Could you check a few things on this model? Use its own coordinates, in mm. Face numbers are marked on the shaded views. A direction names the side the tool comes from. Coordinates: 2 decimals unless noted, no trailing zeros. Loops run counter-clockwise (first coordinate to the right, second up) from the corner with the lowest first, then second, coordinate; pieces in that order, holes last. Notation, with made-up numbers: (3.25, 53.25) -> (57.25, 53.25) arc R4 ccw to (57.25, 59.25) -> close; hole circle Ø2 at (-36, 63). An arc over 180 degrees is marked (long way). One line per question, with ' | ' between items.
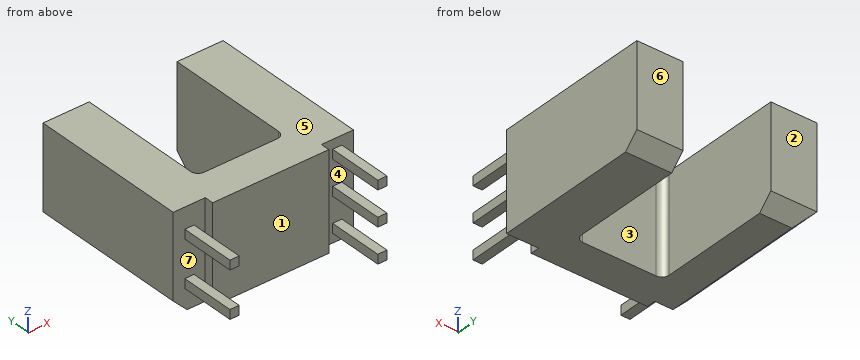
```python
from build123d import *

# Parameters (mm, degrees)
BOSS_EXTRUDE1_DEPTH      = 2.665
CHAMFER1_SIZE            = 0.76
SKETCH2_W                = 1.76
SKETCH2_H                = 5.33
CUT_EXTRUDE1_DEPTH       = 0.5
FILLET1_R                = 0.4
SKETCH3_W                = 0.508
SKETCH3_H                = 0.508
BOSS_EXTRUDE2_DEPTH      = 2.54
BOSS_EXTRUDE2_DEPTH_BACK = 0.5


with BuildPart() as part:
    # Sketch1 → Boss-Extrude1 (new body, symmetric)
    with BuildSketch(Plane.XY):
        Polygon((2.415, 9.27), (4.955, 9.27), (4.955, 0), (-4.955, 0), (-4.955, 9.27), (-2.415, 9.27), (-2.415, 2.03), (2.415, 2.03), align=None)
    extrude(amount=BOSS_EXTRUDE1_DEPTH, both=True)

    # Chamfer1
    chamfer1_edges = [part.edges().sort_by_distance(p)[0] for p in [
        (-4.955, 4.635, -2.665),
        (-3.685, 9.27, -2.665),
        (3.685, 9.27, -2.665),
    ]]
    chamfer(chamfer1_edges, length=CHAMFER1_SIZE)

    # Sketch2 → Cut-Extrude1 (cut)
    with BuildSketch(Plane.XZ):
        with Locations((-4.075, 0)):
            Rectangle(SKETCH2_W, SKETCH2_H)
        with Locations((4.075, 0)):
            Rectangle(SKETCH2_W, SKETCH2_H)
    extrude(amount=-CUT_EXTRUDE1_DEPTH, mode=Mode.SUBTRACT)

    # Fillet1
    fillet1_edges = [part.edges().sort_by_distance(p)[0] for p in [
        (-2.415, 2.03, 0),
        (2.415, 2.03, 0),
    ]]
    fillet(fillet1_edges, radius=FILLET1_R)

    # Sketch3 → Boss-Extrude2 (add, two sides)
    with BuildSketch(Plane.XZ) as boss_extrude2_sk:
        with Locations((4.064, 0)):
            Rectangle(SKETCH3_W, SKETCH3_H)
        with Locations((-4.064, 1.27)):
            Rectangle(SKETCH3_W, SKETCH3_H)
        with Locations((-4.064, -1.27)):
            Rectangle(SKETCH3_W, SKETCH3_H)
        with Locations((4.064, 1.905)):
            Rectangle(SKETCH3_W, SKETCH3_H)
        with Locations((4.064, -1.905)):
            Rectangle(SKETCH3_W, SKETCH3_H)
    extrude(amount=BOSS_EXTRUDE2_DEPTH)
    extrude(boss_extrude2_sk.sketch, amount=-BOSS_EXTRUDE2_DEPTH_BACK)


solid = part.part
```
Q1. Imagine slicing it at B-B on y = 7. Write out the boundary of the cut face in (x, z) (3 decimals), plus the area to 3 significant figures.
Values follow:
outline: (-4.955, -1.905) -> (-4.195, -2.665) -> (-2.415, -2.665) -> (-2.415, 2.665) -> (-4.955, 2.665) -> close; (2.415, -2.665) -> (4.955, -2.665) -> (4.955, 2.665) -> (2.415, 2.665) -> close | area: 26.8 mm2
Q2. Imagine slicing it at C-C on z = 0.45. Write out the boundary of the cut face in (x, y) (3 decimals).
Values follow:
outline: (-4.955, 0.5) -> (-3.195, 0.5) -> (-3.195, 0) -> (3.195, 0) -> (3.195, 0.5) -> (4.955, 0.5) -> (4.955, 9.27) -> (2.415, 9.27) -> (2.415, 2.43) arc R0.4 cw to (2.015, 2.03) -> (-2.015, 2.03) arc R0.4 cw to (-2.415, 2.43) -> (-2.415, 9.27) -> (-4.955, 9.27) -> close
Q3. For pin 1 (2.5 mm diameter, centred on x = 1.5, z = -0.5, fed in from -Y), with a flat end and sliding along its axis, tell me the tip position at first contact or that it passes through.
Values follow:
pin 1: stops at y = 0
Q4. For the marked faces 1, 2 and 3, which set-ups out of +Z, -Z, +X, -X, +Y, -Y let a thin tool reach every point of the face, with its end or its side?
Values follow:
face 1: +Z, -Z, -Y | face 2: +Z, -Z, +X, -X, +Y | face 3: +Z, -Z, +Y
Q5. Imagine slicing it at A-A on y = -0.25. Write out the boundary of the cut face in (x, z), plus the area to 3 significant figures.
Values follow:
outline: (-4.32, -1.52) -> (-3.81, -1.52) -> (-3.81, -1.02) -> (-4.32, -1.02) -> close; (-4.32, 1.02) -> (-3.81, 1.02) -> (-3.81, 1.52) -> (-4.32, 1.52) -> close; (3.81, -2.16) -> (4.32, -2.16) -> (4.32, -1.65) -> (3.81, -1.65) -> close; (3.81, -0.25) -> (4.32, -0.25) -> (4.32, 0.25) -> (3.81, 0.25) -> close; (3.81, 1.65) -> (4.32, 1.65) -> (4.32, 2.16) -> (3.81, 2.16) -> close | area: 1.29 mm2
Q6. Imagine slicing it at D-D on x = -3.5. Write out the boundary of the cut face in (y, z) (3 decimals), plus the area to 3 significant figures.
Values follow:
outline: (0.5, -2.665) -> (8.51, -2.665) -> (9.27, -1.905) -> (9.27, 2.665) -> (0.5, 2.665) -> close | area: 46.5 mm2
Q7. Please list where these lines run through material, in increasing order: L1, parallel to Z at x = 4, y = -1.5; L2, parallel to X at y = 7.25, z = -1.25 (3 decimals); L3, parallel to Y at x = 1.5, z = 0.9. Write a range as [from, to].
Values follow:
L1: z = [-2.16, -1.65], [-0.25, 0.25], [1.65, 2.16] | L2: x = [-4.955, -2.415], [2.415, 4.955] | L3: y = [0, 2.03]
Q8. We'd pull the mould along Z, two halves only. Please class the marked faces 4, 5, 6 and 7: released by +Z, released by -Z, zero draft, split by the parting line, or undercut.
Values follow:
face 4: undercut | face 5: released by +Z | face 6: zero draft | face 7: undercut
